Part model, mm, in its own coordinate system. Coordinates: 2 decimals unless noted, no trailing zeros. Loops run counter-clockwise (first coordinate to the right, second up) from the corner with the lowest first, then second, coordinate; pieces in that order, holes last. Notation, with made-up numbers: (-21, 87) - (-6, 87) arc R21 cw to (-6, 112) - close; hole circle Ø4 at (29, 27.25). An arc over 180 degrees is marked (long way). Answer as CSV lines item,"result".
Autodesk Inventor part; units mm, degrees
ref_plane "YZ Plane" through (0, 0, 0) normal (1, 0, 0) x (0, 1, 0)
ref_plane "XZ Plane" through (0, 0, 0) normal (0, 1, 0) x (-1, 0, 0)
ref_plane "XY Plane" through (0, 0, 0) normal (0, 0, 1) x (1, 0, 0)
sketch "Sketch1" plane through (0, 0, 0) normal (0, 0, 1) x (1, 0, 0)
  circle A0 centre (32, -32) radius 4.7
  circle A1 centre (32, -352) radius 4.7
  line L0 (48, -272) -> (48, -398)
  arc A2 (46, -400) -> (48, -398) centre (46, -398) ccw
  line L1 (46, -400) -> (8, -400)
  line L2 (48, 14) -> (48, -112)
  line L3 (8, 16) -> (46, 16)
  arc A3 (48, 14) -> (46, 16) centre (46, 14) ccw
  circle A4 centre (32, -120) radius 1.85
  circle A5 centre (37.6569, -122.3431) radius 1.85
  circle A6 centre (40, -128) radius 1.85
  circle A7 centre (37.6569, -133.6569) radius 1.85
  circle A8 centre (32, -136) radius 1.85
  circle A9 centre (26.3431, -133.6569) radius 1.85
  circle A10 centre (23.8856, -128.1676) radius 1.85
  circle A11 centre (26.3431, -122.3431) radius 1.85
  circle A12 centre (32, -152) radius 1.85
  circle A13 centre (40, -160) radius 1.85
  circle A14 centre (24, -160) radius 1.85
  circle A15 centre (32, -168) radius 1.85
  circle A16 centre (37.6569, -186.3431) radius 1.85
  circle A17 centre (37.6569, -197.6569) radius 1.85
  circle A18 centre (26.3431, -186.3431) radius 1.85
  circle A19 centre (26.3431, -197.6569) radius 1.85
  circle A20 centre (32, -216) radius 1.85
  circle A21 centre (40, -224) radius 1.85
  circle A22 centre (32, -232) radius 1.85
  circle A23 centre (24, -224) radius 1.85
  circle A24 centre (32, -248) radius 1.85
  circle A25 centre (37.6569, -250.3431) radius 1.85
  circle A26 centre (40, -256) radius 1.85
  circle A27 centre (37.6569, -261.6569) radius 1.85
  circle A28 centre (32, -264) radius 1.85
  circle A29 centre (26.3431, -261.6569) radius 1.85
  circle A30 centre (24, -256) radius 1.85
  circle A31 centre (26.3431, -250.3431) radius 1.85
  circle A32 centre (37.6569, -101.6569) radius 1.85
  circle A33 centre (40, -96) radius 1.85
  circle A34 centre (37.6569, -90.3431) radius 1.85
  circle A35 centre (32, -88) radius 1.85
  circle A36 centre (26.3431, -90.3431) radius 1.85
  circle A37 centre (24, -96) radius 1.85
  circle A38 centre (26.3431, -101.6569) radius 1.85
  circle A39 centre (32, -104) radius 1.85
  circle A40 centre (24, -288.0038) radius 1.85
  circle A41 centre (26.3431, -293.6606) radius 1.85
  circle A42 centre (32, -296.0038) radius 1.85
  circle A43 centre (37.6569, -293.6606) radius 1.85
  circle A44 centre (40, -288.0038) radius 1.85
  circle A45 centre (37.6569, -282.3469) radius 1.85
  circle A46 centre (32, -280.0038) radius 1.85
  circle A47 centre (26.3431, -282.3469) radius 1.85
  line L4 (48, -272) -> (46, -272)
  line L5 (46, -112) -> (48, -112)
  line L6 (46, -112) -> (46, -272)
  line L7 (8, -120.2479) -> (8, 16)
  arc A48 (8, -120.2479) -> (-8.4, -144) centre (17, -144) ccw
  line L8 (-8.4, -240) -> (-8.4, -144)
  arc A49 (-8.4, -240) -> (8, -263.7521) centre (17, -240) ccw
  line L9 (8, -400) -> (8, -263.7521)
  point P0 (0, 0)
  point P1 (48, -114.5)
extrude "Extrusion1" add sketch "Sketch1" along normal blind 2
sketch "Sketch4" plane through (0, 0, 0) normal (0, 0, -1) x (-1, 0, 0)
  circle A0 centre (-40, -390.4) radius 1.85
  circle A1 centre (-24, -390.4) radius 1.85
  circle A2 centre (-40, 6.4) radius 1.85
  circle A3 centre (-24, 6.4) radius 1.85
  point P0 (0, 0)
extrude "Extrusion4" cut sketch "Sketch4" against normal through all
properties part number "plate1"
Q1. Saw through at D-D (x = 4). Give the cut face in (y, z).
Results:
outline,"(-261.82, 0) - (-122.18, 0) - (-122.18, 2) - (-261.82, 2) - close"
Q2. Saw through at A-A (y = -352). Give the cut face in (x, z).
Results:
outline,"(8, 0) - (27.3, 0) - (27.3, 2) - (8, 2) - close; (36.7, 0) - (48, 0) - (48, 2) - (36.7, 2) - close"
Q3. Flat gauge pins, fed straight in: pin 1 (3 mm diameter, centred on x = 40, y = -128, fed in from +Z); pin 2 (0.6 mm diameter, centred on y = -324.5, z = 0.5, fed in from -X). Where does each tip first touch, or does it go through?
Results:
pin 1,"passes through"
pin 2,"stops at x = 8"
Q4. Two-plate mould, pull along Y, no slides. Class faces 1 (the face through (28.3, -29.1, 1)), 2 (the face through (-3.78, -254.61, 0.99)), 3 (the face through (30.98, -347.41, 0.99)), 4 (the face through (26, -189, 0)): released by +Y, released by -Y, zero draft, split by the parting line, or undercut.
Results:
face 1,"undercut"
face 2,"released by -Y"
face 3,"undercut"
face 4,"zero draft"
Q5. Wall check: L1, parallel to X at y = -104, z = 0.9; L2, parallel to X at y = -120, z = 1.5; L3, parallel to Y at x = 30, z = 1. Give the ranges that are in metal, low to high.
Results:
L1,"x = 8 to 30.15, 33.85 to 48"
L2,"x = 8 to 30.15, 33.85 to 46"
L3,"y = -400 to -356.25, -347.75 to -36.25, -27.75 to 16"
Q6. Saw through at B-B (z = 1.4). Count the separate pieces of the cut face and the enclosed holes in it, then the cut area to 3 significant figures.
Results:
separate pieces,"1"
enclosed holes,"50"
area,"17,800 mm^2"
Q7. Saw through at C-C (y = -175). Give the cut face in (x, z).
Results:
outline,"(-8.4, 0) - (46, 0) - (46, 2) - (-8.4, 2) - close"
